Read the model definition and answer for the solid it produces. Units are mm, in the model's axes. A direction names the side the tool comes from. Give positions to 0.01 mm unless a question says otherwise; leave off trailing zeros. Write each loop counter-clockwise with the first axis right and the second up, starting at its lowest first coordinate (ties: lowest second). Pieces come first, ordered by that corner, then holes. Notation, with made-up numbers: M 39,38.5 L 58,38.5 A20 ccw 58,56.5 Z; hole C -15.75,14 d7. An arc over 180 degrees is marked long. Use a Markdown table: item, result. Add a question column.
Item 1: Consider probe 1 along Y at (x, z) = (-36.55, -20.5); probe 2 along Y at (x, z) = (-5.45, -20.1); probe 3 along Z at (x, y) = (-9.5, 16.5). Determine where each line is inside the solid, lowest interval first. Write a range as [from, to].
Item 2: A cutting plane is placed at D-D on x = -5.45. Determine the outline of the cut face in (y, z).
Item 3: For faces 1 (the flat face through (-11, 24.5, -21)), 2 (the cylindrical face through (-32, 21, -18)), 3 (the flat face through (-73, 32, -11)), 4 (the cylindrical face through (-89.4, 23.48, -0.83)), determine the directions among +Z, -Z, +X, -X, +Y, -Y from which every point of the face is accessible in a straight line to the end or side of a thin tool.
Item 4: Given P1, Ø0.9, axis at x = -73, z = 11.5, coming from the +Y side; P2, Ø1, axis at y = 7, z = -6, coming from the +X side; P3, Ø10, axis at x = -55.5, y = 27, coming from the -Z side, each flat-ended and moving along its own axis, determine where each tip first touches the part or whether it passes through.
Item 5: The mould has two halves that part along Z. Classify faces 5 (the flat face through (0, 21, 19)), 6 (the flat face through (-54.68, 20.71, -17.84)), 7 (the cylindrical face through (-101.48, 18.07, -1.15)), 8 (the flat face through (-35, 21, -17.2)): pulls with the +Z half, pulls with the -Z half, needs draft (parallel to the pull), parting line crosses it, or undercut.
Item 6: A cutting plane is placed at B-B on x = -75.5. Determine the outline of the cut face in (y, z).
Item 7: A cutting plane is placed at A-A on x = -36.55. Determine the outline of the cut face in (y, z), then the cut area to 3 significant figures.
from build123d import *

# Parameters (mm, degrees)
BOSS_EXTRUDE1_DEPTH = 42
CUT_EXTRUDE2_DEPTH  = 2.2
CUT_EXTRUDE3_DEPTH  = 5
SKETCH7_R           = 1.75
CUT_EXTRUDE5_DEPTH  = 5
SKETCH8_R           = 2.5
BOSS_EXTRUDE2_DEPTH = 15
SKETCH9_R           = 3
BOSS_EXTRUDE3_DEPTH = 14
SKETCH10_R          = 1.5
CUT_EXTRUDE6_DEPTH  = 10
SKETCH11_R          = 5
BOSS_EXTRUDE4_DEPTH = 3
SKETCH12_R          = 3
BOSS_EXTRUDE5_DEPTH = 3


with BuildPart() as part:
    # Sketch1 → Boss-Extrude1 (new body)
    with BuildSketch(Plane(origin=(0, 0, 0), x_dir=(1, 0, 0), z_dir=(0, 1, 0))):
        Polygon((0, 17.2), (-42, 17.2), (-67, 8.6), (-77, 8.6), (-77, -8.6), (-67, -8.6), (-42, -17.2), (0, -17.2), (0, -21.2), (-42, -21.2), (-67, -12.6), (-82, -12.6), (-82, 13.6), (-67, 13.6), (-42, 22.2), (0, 22.2), align=None)
    extrude(amount=BOSS_EXTRUDE1_DEPTH)

    # Sketch3 → Cut-Extrude2 (cut)
    with BuildSketch(Plane.XY.offset(-17.2)):
        with BuildLine():
            Line((-21, 32), (0, 32))
            Line((0, 32), (0, 10))
            Line((0, 10), (-21, 10))
            ThreePointArc((-21, 10), (-32, 21), (-21, 32))
        make_face()
    extrude(amount=-CUT_EXTRUDE2_DEPTH, mode=Mode.SUBTRACT)

    # Sketch4 → Cut-Extrude3 (cut)
    with BuildSketch(Plane.XY.offset(-17.2)):
        with BuildLine():
            Line((-21, 24.5), (0, 24.5))
            Line((0, 24.5), (0, 17.5))
            Line((0, 17.5), (-21, 17.5))
            ThreePointArc((-21, 17.5), (-24.5, 21), (-21, 24.5))
        make_face()
    extrude(amount=-CUT_EXTRUDE3_DEPTH, mode=Mode.SUBTRACT)

    # Sketch7 → Cut-Extrude5 (cut)
    with BuildSketch(Plane(origin=(0, 0, -22.2), x_dir=(-1, 0, 0), z_dir=(0, 0, -1))):
        with Locations((5.45, 36.55)):
            Circle(SKETCH7_R)
        with Locations((36.55, 36.55)):
            Circle(SKETCH7_R)
        with Locations((5.45, 5.45)):
            Circle(SKETCH7_R)
        with Locations((36.55, 5.45)):
            Circle(SKETCH7_R)
    extrude(amount=-CUT_EXTRUDE5_DEPTH, mode=Mode.SUBTRACT)

    # Sketch8 → Boss-Extrude2 (add)
    with BuildSketch(Plane.ZY.offset(82)):
        with Locations((-0.5, 21)):
            Circle(SKETCH8_R)
    extrude(amount=BOSS_EXTRUDE2_DEPTH)

    # Sketch9 → Boss-Extrude3 (add)
    with BuildSketch(Plane(origin=(0, 0, 17.2), x_dir=(-1, 0, 0), z_dir=(0, 0, -1))):
        with Locations((21, 21)):
            Circle(SKETCH9_R)
    extrude(amount=-BOSS_EXTRUDE3_DEPTH)

    # Sketch10 → Cut-Extrude6 (cut)
    with BuildSketch(Plane(origin=(0, 42, 0), x_dir=(1, 0, 0), z_dir=(0, 1, 0))):
        with Locations((-72.845749412, 11.114300727)):
            Circle(SKETCH10_R)
        with Locations((-72.845749412, -10.607252687)):
            Circle(SKETCH10_R)
    extrude(amount=-CUT_EXTRUDE6_DEPTH, mode=Mode.SUBTRACT)

    # Sketch11 → Boss-Extrude4 (add)
    with BuildSketch(Plane.ZY.offset(97)):
        with Locations((-0.5, 21)):
            Circle(SKETCH11_R)
    extrude(amount=BOSS_EXTRUDE4_DEPTH)

    # Sketch12 → Boss-Extrude5 (add)
    with BuildSketch(Plane.ZY.offset(100)):
        with Locations((-0.5, 21)):
            Circle(SKETCH12_R)
    extrude(amount=BOSS_EXTRUDE5_DEPTH)


solid = part.part
Filled in:
| question | item | result |
|---|---|---|
| 1 | probe 1 | [0, 3.7], [7.2, 34.8], [38.3, 42] |
| 1 | probe 2 | [0, 3.7], [7.2, 17.5], [24.5, 34.8], [38.3, 42] |
| 1 | probe 3 | [-22.2, -19.4], [17.2, 21.2] |
| 2 | outline | M 0,-22.2 L 3.7,-22.2 L 3.7,-17.2 L 0,-17.2 Z; M 0,17.2 L 42,17.2 L 42,21.2 L 0,21.2 Z; M 7.2,-22.2 L 17.5,-22.2 L 17.5,-19.4 L 10,-19.4 L 10,-17.2 L 7.2,-17.2 Z; M 24.5,-22.2 L 34.8,-22.2 L 34.8,-17.2 L 32,-17.2 L 32,-19.4 L 24.5,-19.4 Z; M 38.3,-22.2 L 42,-22.2 L 42,-17.2 L 38.3,-17.2 Z |
| 3 | face 1 | -Z, +X |
| 3 | face 2 | +X |
| 3 | face 3 | +Y |
| 3 | face 4 | none |
| 4 | P1 | y = 32 |
| 4 | P2 | x = -77 |
| 4 | P3 | z = -19.28 |
| 5 | face 5 | needs draft |
| 5 | face 6 | pulls with the -Z half |
| 5 | face 7 | parting line crosses it |
| 5 | face 8 | undercut |
| 6 | outline | M 0,-13.6 L 42,-13.6 L 42,-8.6 L 0,-8.6 Z; M 0,8.6 L 42,8.6 L 42,12.6 L 0,12.6 Z |
| 7 | outline | M 0,-22.2 L 3.7,-22.2 L 3.7,-17.2 L 0,-17.2 Z; M 0,17.2 L 42,17.2 L 42,21.2 L 0,21.2 Z; M 7.2,-22.2 L 34.8,-22.2 L 34.8,-17.2 L 7.2,-17.2 Z; M 38.3,-22.2 L 42,-22.2 L 42,-17.2 L 38.3,-17.2 Z |
| 7 | area | 343 mm² |
